Source: CAD feature listing. Evaluate the final solid. Frame: model axes, mm. Face numbers are marked on the shaded views. A direction names the side the tool comes from. Coordinates: 2 decimals unless noted, no trailing zeros. Write each loop counter-clockwise with the first axis right and the second up, starting at its lowest first coordinate (ties: lowest second). Pieces come first, ordered by that corner, then holes. Notation, with made-up numbers: (83.5, 44) -> (119.5, 44) arc R34 ccw to (119.5, 80) -> close; hole circle Ø9 at (38, 25). An arc over 180 degrees is marked (long way). One line per item, written item: value. Start each with the question number.
1. Section query A-A, the plane y = 0. Output: boundary loops of the cut face in (x, z), and give its area (3 significant figures).
2. Access query for the marked faces 1 and 2. Directions: +Z, -Z, +X, -X, +Y, -Y. A direction counts if a zero-diameter tool reaches every point of the face in a straight line with its end or side. Return the directions, or none.
3. Section query C-C, the plane z = -11.75. Output: boundary loops of the cut face in (x, y).
4. Line query: line 1 (X direction, y = -2, z = -1.25); line 2 (Z direction, x = -11, y = 9); line 3 (Y direction, x = -2.5, z = -8.75). Output: solid intervals per line, ascending.
5. First-contact query: P1, Ø6, axis at x = 0, z = -10.5, coming from the -Y side; P2, Ø4, axis at x = -6.5, z = -7, coming from the -Y side; P3, Ø3, axis at y = 2.5, z = -9.5, coming from the -X side. Flat tips, straight axial feed; report the tip coordinate or a pass-through.
from build123d import *

# Parameters (mm, degrees)
SKETCH1_R           = 16.25
BOSS_EXTRUDE1_DEPTH = 9
SKETCH2_R           = 12.5
BOSS_EXTRUDE3_DEPTH = 5.5
SKETCH3_R           = 16.75
BOSS_EXTRUDE4_DEPTH = 1.5


with BuildPart() as part:
    # Sketch1 → Boss-Extrude1 (new body)
    with BuildSketch(Plane.XY):
        Circle(SKETCH1_R)
    extrude(amount=-BOSS_EXTRUDE1_DEPTH)

    # Sketch2 → Boss-Extrude3 (add)
    with BuildSketch(Plane(origin=(0, 0, -9), x_dir=(-1, 0, 0), z_dir=(0, 0, -1))):
        with Locations(Location((0, 0, 0), (0, 0, 180))):
            Circle(SKETCH2_R)
    extrude(amount=BOSS_EXTRUDE3_DEPTH)

    # Sketch3 → Boss-Extrude4 (add)
    with BuildSketch(Plane.XY):
        Circle(SKETCH3_R)
    extrude(amount=-BOSS_EXTRUDE4_DEPTH)

    # Sketch5 → Cut-Revolve4 (revolve, cut)
    with BuildSketch(Plane(origin=(0, 0, 0), x_dir=(0, 0, -1), z_dir=(1, 0, 0)), mode=Mode.PRIVATE) as cut_revolve4_sk:
        with BuildLine():
            Line((0, 13), (-11.197865554, 13))
            Line((-11.197865554, 13), (-11.197865554, 0))
            Line((-11.197865554, 0), (0, 0))
            ThreePointArc((0, 0), (0.714984963, 4.205055913), (2.779581743, 7.9375))
            ThreePointArc((2.779581743, 7.9375), (0.740603193, 10.112311438), (0, 13))
        make_face()
    revolve(cut_revolve4_sk.sketch.rotate(Axis((0, 0, 11.197865554), (0, 0, -1)), 180), axis=Axis((0, 0, 11.197865554), (0, 0, -1)), mode=Mode.SUBTRACT)


solid = part.part
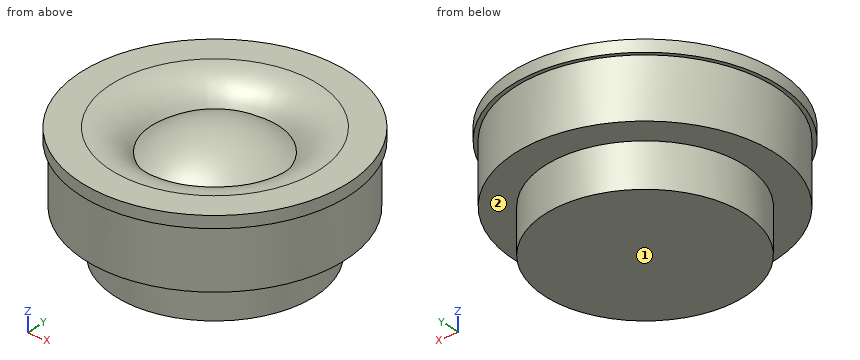
Computed values:
1. outline: (-16.75, -1.5) -> (-16.25, -1.5) -> (-16.25, -9) -> (-12.5, -9) -> (-12.5, -14.5) -> (12.5, -14.5) -> (12.5, -9) -> (16.25, -9) -> (16.25, -1.5) -> (16.75, -1.5) -> (16.75, 0) -> (13, 0) arc R6 ccw to (7.94, -2.78) arc R12.72 ccw to (-7.94, -2.78) arc R6 ccw to (-13, 0) -> (-16.75, 0) -> close
1. area: 409 mm²
2. face 1: -Z, +X, -X, +Y, -Y
2. face 2: -Z
3. outline: circle Ø25 at (0, 0)
4. line 1: x = -16.63 to -9.12, -5.12 to 5.12, 9.12 to 16.63
4. line 2: z = -9 to 0
4. line 3: y = -16.06 to 16.06
5. P1: stops at y = -16.25
5. P2: stops at y = -15.61
5. P3: stops at x = -16.21
